from build123d import *

# Parameters (mm, degrees)
F0_R     = 80
F0_R_2   = 3.1
F0_R_3   = 40
F1_DEPTH = 15


with BuildPart() as f1:
    # F0 (on Front) → F1 (new body)
    with BuildSketch(Plane.XZ):
        Circle(F0_R)
        with Locations((-65, -10)):
            Circle(F0_R_2, mode=Mode.SUBTRACT)
        with Locations((65, -10)):
            Circle(F0_R_2, mode=Mode.SUBTRACT)
        with Locations((-65, 10)):
            Circle(F0_R_2, mode=Mode.SUBTRACT)
        Circle(F0_R_3, mode=Mode.SUBTRACT)
        with Locations((65, 10)):
            Circle(F0_R_2, mode=Mode.SUBTRACT)
    extrude(amount=F1_DEPTH)


solid = f1.part
Input: part model. Units: mm. Frame: model coordinates. Coordinates: 2 decimals unless noted, no trailing zeros. Write each loop counter-clockwise with the first axis right and the second up, starting at its lowest first coordinate (ties: lowest second). Pieces come first, ordered by that corner, then holes. Notation, with made-up numbers: M -27,84 L 21,84 A18 ccw 21,117 Z; hole C 3.25,-39.75 d8. An arc over 180 degrees is marked long. Answer as a JSON object with one key per item and string values. Group by question number.
(1) Section A-A on x = 0. Output: boundary loops of the cut face in (y, z).
(2) Section D-D on x = -65. Output: boundary loops of the cut face in (y, z).
(3) Mould query, pull axis X, two halves, no side actions, for faces 1 (the face through (-37, -15, -17)), 2 (the face through (-17.34, -7.4, -78.1)), 3 (the face through (-62.136, -7.395, 8.813)). Classes: pulls with the +X half, pulls with the -X half, needs draft (parallel to the pull), parting line crosses it, or undercut.
(4) Section B-B on z = 0. Output: boundary loops of the cut face in (x, y), plus the area to 3 significant figures.
(5) Contact query for flat-ended pins moving along their axis: P1, Ø3, axis at x = 40.5, z = 54, coming from the +Y side; P2, Ø5, axis at y = -10, z = 21, coming from the -X side; P3, Ø1.5, axis at y = -2, z = 63, coming from the +X side; P4, Ø10, axis at x = -23, z = 22.5, coming from the -Y side. Output: stop coordinate, or through.
(6) Section C-C on y = -3.5. Output: boundary loops of the cut face in (x, z).
(7) Ray query, line 1 along Z through (x, y) = (65, -3); line 2 along Z through (x, y) = (-27, -1.75); line 3 along Z through (x, y) = (34, -2.5). Return the intervals inside material, ascending. Write a range as [from, to].
Result set:
{
 "1": {"outline": "M -15,-80 L 0,-80 L 0,-40 L -15,-40 Z; M -15,40 L 0,40 L 0,80 L -15,80 Z"},
 "2": {"outline": "M -15,-46.64 L 0,-46.64 L 0,-13.1 L -15,-13.1 Z; M -15,-6.9 L 0,-6.9 L 0,6.9 L -15,6.9 Z; M -15,13.1 L 0,13.1 L 0,46.64 L -15,46.64 Z"},
 "3": {"face 1": "needs draft", "face 2": "parting line crosses it", "face 3": "undercut"},
 "4": {"outline": "M -80,-15 L -40,-15 L -40,0 L -80,0 Z; M 40,-15 L 80,-15 L 80,0 L 40,0 Z", "area": "1,200 mm2"},
 "5": {"P1": "stops at y = 0", "P2": "stops at x = -77.83", "P3": "stops at x = 50.25", "P4": "passes through"},
 "6": {"outline": "C 0,0 d160; hole C -65,-10 d6.2; hole C -65,10 d6.2; hole C 0,0 d80; hole C 65,-10 d6.2; hole C 65,10 d6.2"},
 "7": {"line 1": "z = [-46.64, -13.1], [-6.9, 6.9], [13.1, 46.64]", "line 2": "z = [-75.31, -29.51], [29.51, 75.31]", "line 3": "z = [-72.42, -21.07], [21.07, 72.42]"}
}
